Check sheet for the modelled part. Datum: model origin and axes. Units: mm. A direction names the side the tool comes from. Round coordinates to 2 decimals unless told otherwise and drop trailing zeros. Write each loop counter-clockwise with the first axis right and the second up, starting at its lowest first coordinate (ties: lowest second). Pieces come first, ordered by that corner, then holes.
Item 1: Section check C-C, the plane y = 154. Record the cut outline in (x, z).
Item 2: Section check A-A, the plane z = 0. Record the cut outline in (x, y), plus the area to 3 significant figures.
Item 3: Section check B-B, the plane x = 0. Record the cut outline in (y, z).
Item 4: Material ranges on line 1 along Y through (x, z) = (4, -12.5); line 2 along X through (y, z) = (229, 17); line 3 along X through (y, z) = (168.5, -6), recorded low to high.
Item 5: Depth check by flat-ended pin: pin 1 (6 mm diameter, centred on y = 196.5, z = -13, fed in from -X); pin 2 (10 mm diameter, centred on x = -14.5, y = 90.5, fed in from +Z); pin 3 (12 mm diameter, centred on x = 0.5, y = 45.5, fed in from -Z); pin 4 (10 mm diameter, centred on x = -9.5, z = 9.5, fed in from -Y). Enter the tip coordinate at first touch or a pass-through.
Item 6: Set-up check for faces 1 (the flat face through (0, 310.5, 0)), 2 (the flat face through (-3, 304, 10)), 3 (the cylindrical face through (-2.17, -3.2, -9.76)): record each of +Z, -Z, +X, -X, +Y, -Y from which the full face is reachable in a straight line by a thin tool's end or side.
from build123d import *

# Parameters (mm, degrees)
F0_R     = 10
F1_DEPTH = 6.5
F2_R     = 19
F3_DEPTH = 304
F4_R     = 10
F5_DEPTH = 6.5
F7_R     = 5


with BuildPart() as f1:
    # F0 (on Front) → F1 (new body)
    with BuildSketch(Plane.XZ):
        Circle(F0_R)
    extrude(amount=F1_DEPTH)

    # F2 (on Front) → F3 (join)
    with BuildSketch(Plane.XZ):
        Circle(F2_R)
    extrude(amount=-F3_DEPTH)

    # F4 (on face) → F5 (join)
    with BuildSketch(Plane(origin=(0, 304, 0), x_dir=(-1, 0, 0), z_dir=(0, 1, 0))):
        Circle(F4_R)
    extrude(amount=F5_DEPTH)

    # F7
    f7_edges = [f1.edges().sort_by_distance(p)[0] for p in [
        (-19, 304, 0),
        (-19, 0, 0),
    ]]
    fillet(f7_edges, radius=F7_R)


solid = f1.part
Values found:
1. outline: circle Ø38 at (0, 0)
2. outline: (-19, 5) arc R5 ccw to (-14, 0) - (-10, 0) - (-10, -6.5) - (10, -6.5) - (10, 0) - (14, 0) arc R5 ccw to (19, 5) - (19, 299) arc R5 ccw to (14, 304) - (10, 304) - (10, 310.5) - (-10, 310.5) - (-10, 304) - (-14, 304) arc R5 ccw to (-19, 299) - close
2. area: 11,800 mm2
3. outline: (-6.5, -10) - (0, -10) - (0, -14) arc R5 ccw to (5, -19) - (299, -19) arc R5 ccw to (304, -14) - (304, -10) - (310.5, -10) - (310.5, 10) - (304, 10) - (304, 14) arc R5 ccw to (299, 19) - (5, 19) arc R5 ccw to (0, 14) - (0, 10) - (-6.5, 10) - close
4. line 1: y = 0 to 304
4. line 2: x = -8.49 to 8.49
4. line 3: x = -18.03 to 18.03
5. pin 1: stops at x = -16.16
5. pin 2: stops at z = 16.45
5. pin 3: stops at z = -19
5. pin 4: stops at y = -6.5
6. face 1: +Z, -Z, +X, -X, +Y
6. face 2: +Y
6. face 3: -Y
